For this review, use the dimensioned drawing (mm, ordinates from the lowest corner) and the shaded views. A direction names the side the tool comes from. Coordinates: 2 decimals unless noted, no trailing zeros. Loops run counter-clockwise (first coordinate to the right, second up) from the corner with the lowest first, then second, coordinate; pieces in that order, holes last. Notation, with made-up numbers: (75, -34) - (105, -34) arc R11 cw to (105, -24) - close; hole circle Ø10 at (-32, 34). An arc over 180 degrees is marked (long way). Answer in a Markdown table with one row per item. Add a question column.
(1) To check wall thickness, follow L1, parallel to X at y = 3.35, z = 22 (1 decimal); L2, parallel to Z at x = 21, y = 0.75 (1 decimal); L3, parallel to X at y = 0.6, z = 4.5 (1 decimal). State the ranges of each line that lie inside material, in increasing order. Write a range as [from, to].
(2) We need section C-C, the plane z = 30.75. Give the number of separate pieces and of enclosed holes in the cut face.
(3) We need section A-A, the plane z = 22. Write out the cut boundary in (x, y) (1 decimal).
(4) For the marked faces 1 and 2, list the 3-axis set-ups (+Z, -Z, +X, -X, +Y, -Y) from which the entire face can be reached by the end or side of a thin tool; tool diameter is ignored.
(5) We need section B-B, the plane x = 4.5. Write out the cut boundary in (y, z).
(6) Clearance check with flat-ended pins moving along their axes: pin 1 (1.1 mm diameter, centred on y = 0.5, z = 8.5, fed in from +X) (1 decimal); pin 2 (2 mm diameter, centred on y = 3.5, z = 21.5, fed in from -X) (1 decimal); pin 3 (4.5 mm diameter, centred on x = 20, z = 4, fed in from +Y). State where each tip first meets the part, or that it passes through.
(7) The part is to be moulded in two halves that separate along X. For the marked faces 3 and 4, say which applies: released by +X, released by -X, zero draft, split by the parting line, or undercut.
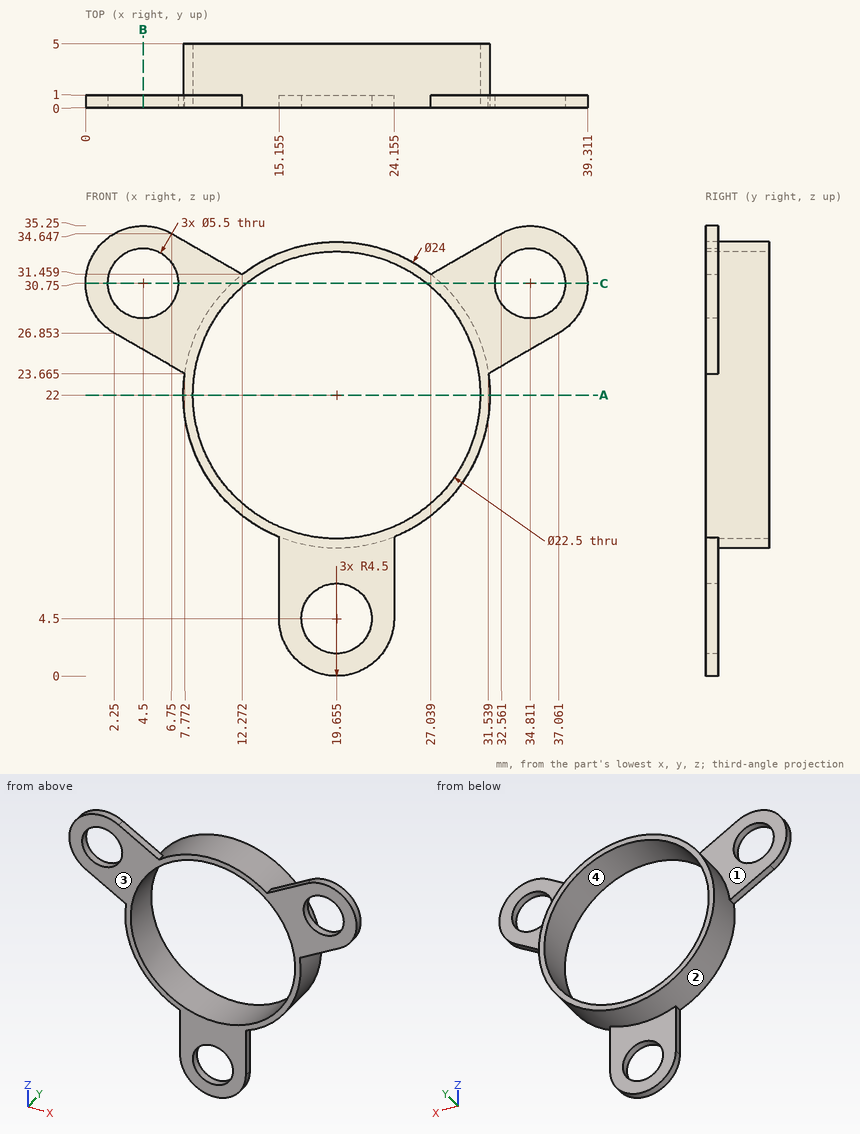
Responses:
| question | item | result |
|---|---|---|
| 1 | L1 | x = [7.7, 8.4], [30.9, 31.7] |
| 1 | L2 | z = [0.2, 2.1], [6.9, 10.8], [33.2, 33.9] |
| 1 | L3 | x = [15.2, 16.9], [22.4, 24.2] |
| 2 | separate pieces | 4 |
| 2 | enclosed holes | 0 |
| 3 | outline | (7.7, 0) - (8.4, 0) - (8.4, 5) - (7.7, 5) - close; (30.9, 0) - (31.7, 0) - (31.7, 5) - (30.9, 5) - close |
| 4 | face 1 | +Z, -X, +Y |
| 4 | face 2 | +Y |
| 5 | outline | (0, 25.55) - (1, 25.55) - (1, 28) - (0, 28) - close; (0, 33.5) - (1, 33.5) - (1, 35.25) - (0, 35.25) - close |
| 6 | pin 1 | stops at x = 24.2 |
| 6 | pin 2 | stops at x = 7.7 |
| 6 | pin 3 | stops at y = 1 |
| 7 | face 3 | zero draft |
| 7 | face 4 | undercut |
